from build123d import *

# Parameters (mm, degrees)
SKETCH1_R           = 34.036
SKETCH1_R_2         = 1.524
SKETCH1_R_3         = 3.302
BOSS_EXTRUDE1_DEPTH = 6.35
CHAMFER1_SIZE       = 1.905
SKETCH2_R           = 1.1303
CUT_EXTRUDE1_DEPTH  = 12.7


with BuildPart() as part:
    # Sketch1 → Boss-Extrude1 (new body)
    with BuildSketch(Plane(origin=(0, 0, 0), x_dir=(1, 0, 0), z_dir=(0, 1, 0))):
        with BuildLine():
            Line((-48.464441263, 25.473804408), (-67.194964824, 28.947993109))
            Line((-67.194964824, 28.947993109), (-68.353027724, 22.704485256))
            Line((-68.353027724, 22.704485256), (-87.083551285, 26.178673957))
            Line((-87.083551285, 26.178673957), (-85.925488385, 32.42218181))
            Line((-85.925488385, 32.42218181), (-104.656011946, 35.896370512))
            Line((-104.656011946, 35.896370512), (-123.386535507, 39.370559213))
            Line((-123.386535507, 39.370559213), (-143.61245558, 43.122118146))
            Line((-143.61245558, 43.122118146), (-173.397808446, 32.12688033))
            Line((-173.397808446, 32.12688033), (-164.230158466, -34.209448348))
            Line((-164.230158466, -34.209448348), (-143.692879271, -77.813892282))
            Line((-143.692879271, -77.813892282), (-76.563330949, -77.813892282))
            Line((-76.563330949, -77.813892282), (-49.204879271, -77.813892282))
            Line((-49.204879271, -77.813892282), (-49.204879271, -37.681892282))
            Line((-49.204879271, -37.681892282), (45.277962712, -37.681892282))
            Line((45.277962712, -37.681892282), (64.72671994, -37.681892282))
            ThreePointArc((64.72671994, -37.681892282), (47.456106683, -24.721818432), (40.256527969, -4.364911427))
            ThreePointArc((40.256527969, -4.364911427), (40.224315343, -2.464216219), (40.304028245, -0.564920092))
            ThreePointArc((40.304028245, -0.564920092), (40.358687129, 0.79375425), (40.328560009, 2.153193811))
            ThreePointArc((40.328560009, 2.153193811), (38.274981353, 12.886225143), (33.41911498, 22.675796567))
            ThreePointArc((33.41911498, 22.675796567), (30.929713329, 27.951337515), (30.171477502, 33.73524029))
            ThreePointArc((30.171477502, 33.73524029), (27.651370412, 37.853265988), (22.862043617, 37.243820127))
            ThreePointArc((22.862043617, 37.243820127), (20.166682607, 36.055874133), (17.256896531, 36.513401897))
            ThreePointArc((17.256896531, 36.513401897), (8.843040964, 39.405959226), (0, 40.386))
            ThreePointArc((0, 40.386), (-9.489488111, 40.375548652), (-18.94466273, 39.569219451))
            ThreePointArc((-18.94466273, 39.569219451), (-22.43398811, 39.812343861), (-25.563809609, 41.373983535))
            ThreePointArc((-25.563809609, 41.373983535), (-32.045487778, 43.349075748), (-38.20024979, 40.514989348))
            ThreePointArc((-38.20024979, 40.514989348), (-40.697264896, 36.549064779), (-41.325740518, 31.904857578))
            ThreePointArc((-41.325740518, 31.904857578), (-43.308574881, 26.928241056), (-48.464441263, 25.473804408))
        make_face()
        with Locations(Location((0, 0, 0), (0, 0, 270))):
            Circle(SKETCH1_R, mode=Mode.SUBTRACT)
        with Locations(Location((-31.399492492, 33.846007028, 0), (0, 0, 270))):
            Circle(SKETCH1_R_2, mode=Mode.SUBTRACT)
        with Locations(Location((-74.604879271, -57.747892282, 0), (0, 0, 270))):
            Circle(SKETCH1_R_3, mode=Mode.SUBTRACT)
        with Locations(Location((-40.020695033, -13.367428306, 0), (0, 0, 270))):
            Circle(SKETCH1_R_2, mode=Mode.SUBTRACT)
        with Locations(Location((-131.808500509, 37.703534036, 0), (0, 0, 270))):
            Circle(SKETCH1_R_2, mode=Mode.SUBTRACT)
        with Locations(Location((25.727857837, 33.846007028, 0), (0, 0, 270))):
            Circle(SKETCH1_R_2, mode=Mode.SUBTRACT)
        with BuildLine():
            Line((-142.716614997, 32.622661546), (-162.215024971, 25.424839997))
            Line((-162.215024971, 25.424839997), (-156.726187502, -14.291916989))
            ThreePointArc((-156.726187502, -14.291916989), (-128.010283659, 5.891204619), (-94.602827713, 16.657049623))
            ThreePointArc((-94.602827713, 16.657049623), (-91.648252867, 20.09262068), (-94.526212577, 23.592621954))
            Line((-94.526212577, 23.592621954), (-142.716614997, 32.622661546))
        make_face(mode=Mode.SUBTRACT)
        with BuildLine():
            Line((-114.508797405, -72.415483536), (-119.588797405, -72.415483536))
            ThreePointArc((-119.588797405, -72.415483536), (-124.351297405, -67.652983536), (-119.588797405, -62.890483536))
            Line((-119.588797405, -62.890483536), (-114.508797405, -62.890483536))
            ThreePointArc((-114.508797405, -62.890483536), (-109.746297405, -67.652983536), (-114.508797405, -72.415483536))
        make_face(mode=Mode.SUBTRACT)
        with BuildLine():
            ThreePointArc((-147.948535824, -23.470306336), (-122.347176599, -5.47625853), (-92.563113904, 4.121916294))
            ThreePointArc((-92.563113904, 4.121916294), (-89.845720269, 1.990682905), (-91.74722838, -0.892137038))
            ThreePointArc((-91.74722838, -0.892137038), (-120.081933775, -10.023243789), (-144.437475152, -27.141662075))
            ThreePointArc((-144.437475152, -27.141662075), (-147.689154448, -26.736809805), (-147.948535824, -23.470306336))
        make_face(mode=Mode.SUBTRACT)
    extrude(amount=BOSS_EXTRUDE1_DEPTH)

    # Chamfer1
    # the kernel refuses this chamfer: 1.905 mm, written as the material it takes off along each edge
    with BuildSketch(Plane(origin=(-40.020695033, 6.35, 13.367428306), x_dir=(0, 0, 1), z_dir=(-1, 0, 0))) as chamfer1_piece_1:
        Polygon((1.524 + CHAMFER1_SIZE, 0), (1.524, -CHAMFER1_SIZE), (1.524, 0), align=None)
    revolve(axis=Axis((-40.020695033, 6.35, 13.367428306), (0, 1, 0)), mode=Mode.SUBTRACT)
    with BuildSketch(Plane(origin=(-131.808500509, 6.35, -37.703534036), x_dir=(0, 0, 1), z_dir=(-1, 0, 0))) as chamfer1_piece_2:
        Polygon((1.524 + CHAMFER1_SIZE, 0), (1.524, -CHAMFER1_SIZE), (1.524, 0), align=None)
    revolve(axis=Axis((-131.808500509, 6.35, -37.703534036), (0, 1, 0)), mode=Mode.SUBTRACT)
    with BuildSketch(Plane(origin=(25.727857837, 6.35, -33.846007028), x_dir=(0, 0, 1), z_dir=(-1, 0, 0))) as chamfer1_piece_3:
        Polygon((1.524 + CHAMFER1_SIZE, 0), (1.524, -CHAMFER1_SIZE), (1.524, 0), align=None)
    revolve(axis=Axis((25.727857837, 6.35, -33.846007028), (0, 1, 0)), mode=Mode.SUBTRACT)
    with BuildSketch(Plane(origin=(-31.399492492, 6.35, -33.846007028), x_dir=(0, 0, 1), z_dir=(-1, 0, 0))) as chamfer1_piece_4:
        Polygon((1.524 + CHAMFER1_SIZE, 0), (1.524, -CHAMFER1_SIZE), (1.524, 0), align=None)
    revolve(axis=Axis((-31.399492492, 6.35, -33.846007028), (0, 1, 0)), mode=Mode.SUBTRACT)

    # Sketch2 → Cut-Extrude1 (cut)
    with BuildSketch(Plane(origin=(1.797830768, 0, -9.692712298), x_dir=(-0.9832295832535878, 0, -0.18237211029917974), z_dir=(0.18237211029917974, 0, -0.9832295832535878))):
        with Locations((80.872383853, 3.175)):
            Circle(SKETCH2_R)
    extrude(amount=-CUT_EXTRUDE1_DEPTH, mode=Mode.SUBTRACT)


solid = part.part
Design review of the part built by this model. Coordinates are the model's own, in mm. A direction names the side the tool comes from. Give positions to 0.01 mm unless a question says otherwise; leave off trailing zeros. Order: outer loops, then holes, each group sorted by start corner. A loop starts at its lowest first (then second) coordinate and runs counter-clockwise, first axis right, second up. Notation, with made-up numbers: (31.25, 26) - (71.25, 26) arc R21 cw to (71.25, 30) - close; hole circle Ø3 at (-25.75, 13). An arc over 180 degrees is marked (long way). Use CSV: the item, a comma, the result in double quotes. Start each with the question number.
Q1. Take a section at A-A (z = 30). State the section outline as (x, y) points, and give its area (3 significant figures).
Q2. Draft analysis for pull direction X (two halves, no side actions). For faces 4 (the face through (7, 3, 37.682)), 5 (the face through (-49.205, 3, 58)), 6 (the face through (-152.329, 3.131, -29.074)), state which applies: pulls with the +X half, pulls with the -X half, needs draft (parallel to the pull), parting line crosses it, or undercut.
Q3. Machinability: for faces 1 (the face through (-57.699, 3.131, -27.187)), 2 (the face through (-117, 3, 62.89)), 3 (the face through (-82, 6.35, 16)), which of the approach directions +Z, -Z, +X, -X, +Y, -Y give a long, thin tool a straight path to every point of the face, cutting with its end or side? Answer none if there is none.
Q4. For line 1 (Z direction, x = -116.5, y = 3); line 2 (Z direction, x = -127.5, y = 3.75); line 3 (X direction, y = 1.75, z = 8.5), list the stretches that pass through material, from the lowest coordinate up.
Q5. For P1, Ø4, axis at x = -40.02, z = 13.37, coming from the -Y side; P2, Ø3, axis at x = 22, y = 3.5, coming from the +Z side; P3, Ø3, axis at y = 5.5, z = 14, coming from the +X side; P4, Ø2, axis at x = -134, y = 5.5, coming from the -Z side, all flat-tipped, find the tip position at first contact; note any pin that passes through.
Calculated:
1,outline,"(-164.81, 0) - (-16.08, 0) - (-16.08, 6.35) - (-164.81, 6.35) - close; (16.08, 0) - (52.16, 0) - (52.16, 6.35) - (16.08, 6.35) - close"
1,area,"1,170 mm²"
2,face 4,"needs draft"
2,face 5,"pulls with the +X half"
2,face 6,"undercut"
3,face 1,"-Z, +Y, -Y"
3,face 2,"+Y, -Y"
3,face 3,"+Z, -Z, +X, -X, +Y"
4,line 1,"z = -38.09 to -27.71, -10.87 to 2.78, 8.33 to 62.89, 72.42 to 77.81"
4,line 2,"z = -40.13 to -29.77, -6.14 to 8.23, 14.12 to 77.81"
4,line 3,"x = -167.78 to -157.53, -150.2 to -127.98, -116.88 to -32.96, 32.96 to 40.68"
5,P1,"stops at y = 0"
5,P2,"stops at z = 37.68"
5,P3,"stops at x = 42.5"
5,P4,"stops at z = -41.52"
